Geometry: final body of the model. Coordinates: model frame, mm. A direction names the side the tool comes from. Coordinates: 2 decimals unless noted, no trailing zeros. Loops run counter-clockwise (first coordinate to the right, second up) from the corner with the lowest first, then second, coordinate; pieces in that order, holes last. Notation, with made-up numbers: (84, 87) - (88, 87) arc R23 ccw to (88, 97) - close; hole circle Ø8 at (-28, 87). An arc over 180 degrees is marked (long way). Return JSON: item names as keys, results as strings.
from build123d import *

# Parameters (mm, degrees)
BOSS_EXTRUDE1_DEPTH = 196
CUT_EXTRUDE4_REACH  = 17
SKETCH5_R           = 2.25
CUT_EXTRUDE5_REACH  = 14
SKETCH6_R           = 2.25


with BuildPart() as part:
    # Sketch1 → Boss-Extrude1 (new body)
    with BuildSketch(Plane(origin=(0, 0, 0), x_dir=(1, 0, 0), z_dir=(0, 1, 0))):
        Polygon((0, 0), (15, 0), (15, 12), (14.5, 12), (14.5, 0.5), (0, 0.5), align=None)
    extrude(amount=BOSS_EXTRUDE1_DEPTH)

    # Sketch5 → Cut-Extrude4 (cut, up to next)
    with BuildSketch(Plane(origin=(15, 0, 0), x_dir=(0, 0, -1), z_dir=(1, 0, 0)), mode=Mode.PRIVATE) as cut_extrude4_sk1:
        with Locations((4.5, 23)):
            Circle(SKETCH5_R)
    cut_extrude4_tool1 = extrude(cut_extrude4_sk1.sketch, amount=-CUT_EXTRUDE4_REACH, mode=Mode.PRIVATE) & part.part
    add(cut_extrude4_tool1.solids().sort_by_distance((15, 23, -4.5))[0], mode=Mode.SUBTRACT)
    # Sketch5 → Cut-Extrude4 (cut, up to next)
    with BuildSketch(Plane(origin=(15, 0, 0), x_dir=(0, 0, -1), z_dir=(1, 0, 0)), mode=Mode.PRIVATE) as cut_extrude4_sk2:
        with Locations((4.5, 55.5)):
            Circle(SKETCH5_R)
    cut_extrude4_tool2 = extrude(cut_extrude4_sk2.sketch, amount=-CUT_EXTRUDE4_REACH, mode=Mode.PRIVATE) & part.part
    add(cut_extrude4_tool2.solids().sort_by_distance((15, 55.5, -4.5))[0], mode=Mode.SUBTRACT)
    # Sketch5 → Cut-Extrude4 (cut, up to next)
    with BuildSketch(Plane(origin=(15, 0, 0), x_dir=(0, 0, -1), z_dir=(1, 0, 0)), mode=Mode.PRIVATE) as cut_extrude4_sk3:
        with Locations((4.5, 88)):
            Circle(SKETCH5_R)
    cut_extrude4_tool3 = extrude(cut_extrude4_sk3.sketch, amount=-CUT_EXTRUDE4_REACH, mode=Mode.PRIVATE) & part.part
    add(cut_extrude4_tool3.solids().sort_by_distance((15, 88, -4.5))[0], mode=Mode.SUBTRACT)
    # Sketch5 → Cut-Extrude4 (cut, up to next)
    with BuildSketch(Plane(origin=(15, 0, 0), x_dir=(0, 0, -1), z_dir=(1, 0, 0)), mode=Mode.PRIVATE) as cut_extrude4_sk4:
        with Locations((4.5, 108)):
            Circle(SKETCH5_R)
    cut_extrude4_tool4 = extrude(cut_extrude4_sk4.sketch, amount=-CUT_EXTRUDE4_REACH, mode=Mode.PRIVATE) & part.part
    add(cut_extrude4_tool4.solids().sort_by_distance((15, 108, -4.5))[0], mode=Mode.SUBTRACT)
    # Sketch5 → Cut-Extrude4 (cut, up to next)
    with BuildSketch(Plane(origin=(15, 0, 0), x_dir=(0, 0, -1), z_dir=(1, 0, 0)), mode=Mode.PRIVATE) as cut_extrude4_sk5:
        with Locations((4.5, 140.5)):
            Circle(SKETCH5_R)
    cut_extrude4_tool5 = extrude(cut_extrude4_sk5.sketch, amount=-CUT_EXTRUDE4_REACH, mode=Mode.PRIVATE) & part.part
    add(cut_extrude4_tool5.solids().sort_by_distance((15, 140.5, -4.5))[0], mode=Mode.SUBTRACT)
    # Sketch5 → Cut-Extrude4 (cut, up to next)
    with BuildSketch(Plane(origin=(15, 0, 0), x_dir=(0, 0, -1), z_dir=(1, 0, 0)), mode=Mode.PRIVATE) as cut_extrude4_sk6:
        with Locations((4.5, 173)):
            Circle(SKETCH5_R)
    cut_extrude4_tool6 = extrude(cut_extrude4_sk6.sketch, amount=-CUT_EXTRUDE4_REACH, mode=Mode.PRIVATE) & part.part
    add(cut_extrude4_tool6.solids().sort_by_distance((15, 173, -4.5))[0], mode=Mode.SUBTRACT)

    # Sketch6 → Cut-Extrude5 (cut, up to next)
    with BuildSketch(Plane.XY, mode=Mode.PRIVATE) as cut_extrude5_sk1:
        with Locations((7.5, 23.833333333)):
            Circle(SKETCH6_R)
    cut_extrude5_tool1 = extrude(cut_extrude5_sk1.sketch, amount=-CUT_EXTRUDE5_REACH, mode=Mode.PRIVATE) & part.part
    add(cut_extrude5_tool1.solids().sort_by_distance((7.5, 23.833333, 0))[0], mode=Mode.SUBTRACT)
    # Sketch6 → Cut-Extrude5 (cut, up to next)
    with BuildSketch(Plane.XY, mode=Mode.PRIVATE) as cut_extrude5_sk2:
        with Locations((7.5, 57.166666667)):
            Circle(SKETCH6_R)
    cut_extrude5_tool2 = extrude(cut_extrude5_sk2.sketch, amount=-CUT_EXTRUDE5_REACH, mode=Mode.PRIVATE) & part.part
    add(cut_extrude5_tool2.solids().sort_by_distance((7.5, 57.166667, 0))[0], mode=Mode.SUBTRACT)
    # Sketch6 → Cut-Extrude5 (cut, up to next)
    with BuildSketch(Plane.XY, mode=Mode.PRIVATE) as cut_extrude5_sk3:
        with Locations((7.5, 90.5)):
            Circle(SKETCH6_R)
    cut_extrude5_tool3 = extrude(cut_extrude5_sk3.sketch, amount=-CUT_EXTRUDE5_REACH, mode=Mode.PRIVATE) & part.part
    add(cut_extrude5_tool3.solids().sort_by_distance((7.5, 90.5, 0))[0], mode=Mode.SUBTRACT)
    # Sketch6 → Cut-Extrude5 (cut, up to next)
    with BuildSketch(Plane.XY, mode=Mode.PRIVATE) as cut_extrude5_sk4:
        with Locations((7.5, 105.5)):
            Circle(SKETCH6_R)
    cut_extrude5_tool4 = extrude(cut_extrude5_sk4.sketch, amount=-CUT_EXTRUDE5_REACH, mode=Mode.PRIVATE) & part.part
    add(cut_extrude5_tool4.solids().sort_by_distance((7.5, 105.5, 0))[0], mode=Mode.SUBTRACT)
    # Sketch6 → Cut-Extrude5 (cut, up to next)
    with BuildSketch(Plane.XY, mode=Mode.PRIVATE) as cut_extrude5_sk5:
        with Locations((7.5, 138.833333333)):
            Circle(SKETCH6_R)
    cut_extrude5_tool5 = extrude(cut_extrude5_sk5.sketch, amount=-CUT_EXTRUDE5_REACH, mode=Mode.PRIVATE) & part.part
    add(cut_extrude5_tool5.solids().sort_by_distance((7.5, 138.833333, 0))[0], mode=Mode.SUBTRACT)
    # Sketch6 → Cut-Extrude5 (cut, up to next)
    with BuildSketch(Plane.XY, mode=Mode.PRIVATE) as cut_extrude5_sk6:
        with Locations((7.5, 172.166666667)):
            Circle(SKETCH6_R)
    cut_extrude5_tool6 = extrude(cut_extrude5_sk6.sketch, amount=-CUT_EXTRUDE5_REACH, mode=Mode.PRIVATE) & part.part
    add(cut_extrude5_tool6.solids().sort_by_distance((7.5, 172.166667, 0))[0], mode=Mode.SUBTRACT)


solid = part.part
Item 1: Section query B-B, the plane x = 7.5. Return loops of the section in (y, z), and give its area (3 significant figures).
Worked out:
{"outline": "(0, -0.5) - (21.58, -0.5) - (21.58, 0) - (0, 0) - close; (26.08, -0.5) - (54.92, -0.5) - (54.92, 0) - (26.08, 0) - close; (59.42, -0.5) - (88.25, -0.5) - (88.25, 0) - (59.42, 0) - close; (92.75, -0.5) - (103.25, -0.5) - (103.25, 0) - (92.75, 0) - close; (107.75, -0.5) - (136.58, -0.5) - (136.58, 0) - (107.75, 0) - close; (141.08, -0.5) - (169.92, -0.5) - (169.92, 0) - (141.08, 0) - close; (174.42, -0.5) - (196, -0.5) - (196, 0) - (174.42, 0) - close", "area": "84.5 mm^2"}
Item 2: Section query A-A, the plane z = -4.5. Return loops of the section in (x, y).
Worked out:
{"outline": "(14.5, 0) - (15, 0) - (15, 20.75) - (14.5, 20.75) - close; (14.5, 25.25) - (15, 25.25) - (15, 53.25) - (14.5, 53.25) - close; (14.5, 57.75) - (15, 57.75) - (15, 85.75) - (14.5, 85.75) - close; (14.5, 90.25) - (15, 90.25) - (15, 105.75) - (14.5, 105.75) - close; (14.5, 110.25) - (15, 110.25) - (15, 138.25) - (14.5, 138.25) - close; (14.5, 142.75) - (15, 142.75) - (15, 170.75) - (14.5, 170.75) - close; (14.5, 175.25) - (15, 175.25) - (15, 196) - (14.5, 196) - close"}
Item 3: Section query C-C, the plane y = 40. Return loops of the section in (x, z).
Worked out:
{"outline": "(0, -0.5) - (14.5, -0.5) - (14.5, -12) - (15, -12) - (15, 0) - (0, 0) - close"}
Item 4: Ray query, probe 1 along Z at (x, y) = (14.7, 140.5); probe 2 along X at (y, z) = (18.5, -5.75); probe 3 along Z at (x, y) = (3.5, 115). Return the intervals inside material, ascending. Write a range as from..to.
Worked out:
{"probe 1": "-12..-6.75, -2.25..0", "probe 2": "14.5..15", "probe 3": "-0.5..0"}
Item 5: First-contact query: pin 1 Ø7 at (y, z) = (55.5, -4.5) entering from -X; pin 2 Ø7 at (x, y) = (3.5, 55.5) entering from -Z. Flat tips, straight axial feed; report the tip coordinate or a pass-through.
Worked out:
{"pin 1": "x = 14.5", "pin 2": "z = -0.5"}
Item 6: Mould query, pull axis Z, two halves, no side actions, for faces 1 (the face through (14.754, 138.504, -5.538)), 2 (the face through (7, 97, -0.5)), 3 (the face through (5.714, 170.798, -0.246)), 4 (the face through (7, 97, 0)). Classes: +Z half, -Z half, draft (parallel to the pull), parting line (faces both ways), or undercut.
Worked out:
{"face 1": "undercut", "face 2": "-Z half", "face 3": "draft", "face 4": "+Z half"}
Item 7: Reachability of faces 5 (the face through (7.01, 54.97, -0.25)), 6 (the face through (14.5, 97, -6)) from +Z, -Z, +X, -X, +Y, -Y: full face, straight path, thin tool, end or side. Return the list, or none.
Worked out:
{"face 5": "+Z, -Z", "face 6": "-Z, -X, +Y, -Y"}
